Source: CAD feature listing. Evaluate the final solid. Frame: model axes, mm. A direction names the side the tool comes from. Round coordinates to 2 decimals unless told otherwise and drop trailing zeros. Loops run counter-clockwise (first coordinate to the right, second up) from the corner with the lowest first, then second, coordinate; pieces in that order, holes last. Notation, with made-up numbers: (2, -6.75) -> (21, -6.75) arc R27 ccw to (21, 31.25) -> close; hole circle Ø1 at (45, 75). An arc over 180 degrees is marked (long way). Return JSON: item names as keys, results as strings. Group by question number.
```python
from build123d import *

# Parameters (mm, degrees)
SKETCH_1_W          = 30
SKETCH_1_H          = 30
EXTRUDE_1_DEPTH     = 8
SKETCH_2_R          = 12.45
EXTRUDE_2_DEPTH     = 65
SKETCH_3_W          = 15
SKETCH_3_H          = 30
CUT_EXTRUDE_1_DEPTH = 85.433405711
FILLET_1_R          = 2
FILLET_2_R          = 1


with BuildPart() as part:
    # 草图1 → 凸台-拉伸1 (new body)
    with BuildSketch(Plane(origin=(0, 0, 0), x_dir=(1, 0, 0), z_dir=(0, 1, 0))):
        with Locations((-15, 15)):
            Rectangle(SKETCH_1_W, SKETCH_1_H)
    extrude(amount=EXTRUDE_1_DEPTH)

    # 草图2 → 凸台-拉伸2 (add)
    with BuildSketch(Plane.XZ):
        with Locations(Location((-15, -15, 0), (0, 0, 270))):
            Circle(SKETCH_2_R)
    extrude(amount=EXTRUDE_2_DEPTH)

    # 草图3 → 切除-拉伸1 (cut, through all)
    with BuildSketch(Plane(origin=(0, 8, 0), x_dir=(1, 0, 0), z_dir=(0, 1, 0))):
        with Locations((-22.5, 15)):
            Rectangle(SKETCH_3_W, SKETCH_3_H)
    extrude(amount=-CUT_EXTRUDE_1_DEPTH, mode=Mode.SUBTRACT)

    # 圆角1
    fillet_1_edges = [part.edges().sort_by_distance(p)[0] for p in [
        (-2.55, -65, -15),
    ]]
    fillet(fillet_1_edges, radius=FILLET_1_R)

    # 圆角2
    fillet_2_edges = [part.edges().sort_by_distance(p)[0] for p in [
        (-7.5, 0, 0),
        (-7.5, 8, 0),
        (-15, 4, 0),
        (-15, 4, -30),
        (-7.5, 0, -30),
        (0, 0, -15),
        (0, 4, 0),
        (0, 4, -30),
        (-7.5, 8, -30),
    ]]
    fillet(fillet_2_edges, radius=FILLET_2_R)


solid = part.part
```
(1) Ray query, line 1 (X direction, y = -40.5, z = -8.25); line 2 (Y direction, x = -1.5, z = -20); line 3 (Z direction, x = -7.25, y = -33). Return the intervals inside material, ascending.
(2) Cut plane A-A (z = -15). Return loops of the section in (x, y).
(3) Set-up query: faces 1 (the face through (-2, 0, -15)), 2 (the face through (-8, 4, 0)). Return all of +Z, -Z, +X, -X, +Y, -Y with unobstructed straight access to the full face (end or side cutting, diameter ignored); none if empty.
(4) Cut plane B-B (y = -59.5). Return loops of the section in (x, z).
(5) Pin query (flat end, axial travel): pin 1 (6 mm diameter, centred on y = -19.5, z = -26, fed in from +X); pin 2 (1 mm diameter, centred on x = -9.5, y = -9, fed in from -Z); pin 3 (5 mm diameter, centred on y = -10.5, z = -6, fed in from +X). Return the tip coordinate at first contact, or that it passes through.
Answers follow:
{
 "1": {"line 1": "-15 to -4.54", "line 2": "0 to 8", "line 3": "-24.74 to -5.26"},
 "2": {"outline": "(-15, -65) -> (-4.55, -65) arc R2 ccw to (-2.55, -63) -> (-2.55, 0) -> (-1, 0) arc R1 ccw to (0, 1) -> (0, 8) -> (-15, 8) -> close"},
 "3": {"face 1": "+X, -Y", "face 2": "+Z, +X, -X, +Y, -Y"},
 "4": {"outline": "(-15, -27.45) arc R12.45 ccw to (-15, -2.55) -> close"},
 "5": {"pin 1": "x = -5.46", "pin 2": "z = -26.4", "pin 3": "x = -4.38"}
}
